```python
from build123d import *

# Parameters (mm, degrees)
SKETCH3_R           = 0.6
BOSS_EXTRUDE1_DEPTH = 2.5
CIRPATTERN1_COUNT   = 4
BOSS_EXTRUDE2_DEPTH = 1


with BuildPart() as part:
    # Sketch2 → Revolve1 (revolve)
    with BuildSketch(Plane(origin=(0, 0, 0), x_dir=(0, 0, -1), z_dir=(1, 0, 0))):
        Polygon((0, 8.815), (0, 10), (-1.5, 10), (-1.5, 7.74), (5, 7.74), (5, 5.555), (0.5, 5.555), (0.5, 0), (11.17, 0), (11.17, 7.25), (10.130849194, 7.25), (9, 8.815), align=None)
    revolve(axis=Axis((0, 0, 11.357142857), (0, 0, -1)))

    # Sketch3 → Boss-Extrude1 (add)
    with BuildSketch(Plane(origin=(0, 0, -11.17), x_dir=(-1, 0, 0), z_dir=(0, 0, -1))):
        with Locations((1.71395454, 3.773699623)):
            Circle(SKETCH3_R)
        with Locations((1.71395454, 1.968598852)):
            Circle(SKETCH3_R)
        with Locations((3.52115951, 1.968598852)):
            Circle(SKETCH3_R)
    boss_extrude1 = extrude(amount=BOSS_EXTRUDE1_DEPTH)

    # CirPattern1: Boss-Extrude1 ×4 about axis
    cirpattern1_axis = Axis((0, 0, 0), (0, 0, 1))
    for i in range(1, CIRPATTERN1_COUNT):
        add(boss_extrude1.rotate(cirpattern1_axis, i * 360 / CIRPATTERN1_COUNT))

    # Sketch5 → Boss-Extrude2 (add)
    with BuildSketch(Plane(origin=(0, 0, 0), x_dir=(-1, 0, 0), z_dir=(0, 0, -1))):
        with BuildLine():
            Line((-0.71671494, 9.974282916), (-0.71671494, 8.78581497))
            ThreePointArc((-0.71671494, 8.78581497), (0, 8.815), (0.71671494, 8.78581497))
            Line((0.71671494, 8.78581497), (0.71671494, 9.974282916))
            ThreePointArc((0.71671494, 9.974282916), (0, 10), (-0.71671494, 9.974282916))
        make_face()
    extrude(amount=BOSS_EXTRUDE2_DEPTH)


solid = part.part
```
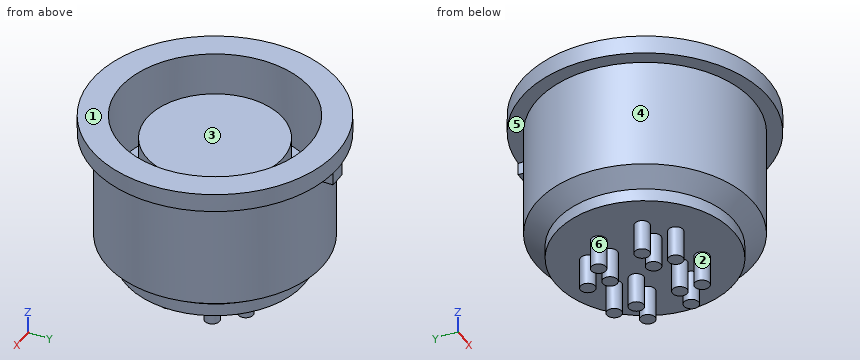
Part model, mm, in its own coordinate system. Face numbers are marked on the shaded views. A direction names the side the tool comes from. Round coordinates to 2 decimals unless told otherwise and drop trailing zeros. Loops run counter-clockwise (first coordinate to the right, second up) from the corner with the lowest first, then second, coordinate; pieces in that order, holes last. Notation, with made-up numbers: (48, 40) -> (58, 40) arc R30 cw to (58, 73) -> close; hole circle Ø4 at (11, 12.5). An arc over 180 degrees is marked (long way). Use one line per item in the form item = value. Start each with the question number.
Item 1: Two-plate mould, pull along Y, no slides. Class the marked faces 4, 5 and 6: released by +Y, released by -Y, zero draft, split by the parting line, or undercut.
Item 2: Band-saw the part on C-C (y = 0). List the corners of the cut face in (x, z) (3 decimals), plus the area to 3 significant figures.
Item 3: Drill centre lines: line 1 along X through (y, z) = (0, -1.75) (3 decimals); line 2 along Z through (x, y) = (-2.75, -1.75); line 3 along X through (y, z) = (-6.75, -3.5). Where is each one in solid material? Low to high.
Item 4: Band-saw the part on A-A (x = 0). List the corners of the cut face in (y, z) (3 decimals), plus the area to 3 significant figures.
Item 5: Band-saw the part on D-D (z = -11.5). Give the number of separate pieces and of enclosed holes in the cut face, plus the area to 3 significant figures.
Item 6: Tool access for the marked faces 1, 2 and 3: list every direction of +Z, -Z, +X, -X, +Y, -Y with a clear straight run to the whole face (end or side of a thin tool).
Item 7: Band-saw the part on B-B (z = -2.5). List the corners of the cut face in (x, y) (3 decimals), plus the area to 3 significant figures.
Item 8: Drop flat-ended pins along their axis: pin 1 Ø3 at (x, z) = (-2, -1) entering from -Y; pin 2 Ø1 at (y, z) = (-4.5, -9) entering from +X; pin 3 Ø10 at (x, y) = (-6, 2.5) entering from +Z; pin 4 Ø12 at (x, y) = (1, 1) entering from +Z. Give the stop position or say it passes through.
Data:
q1.face_4 = split by the parting line
q1.face_5 = zero draft
q1.face_6 = undercut
q2.outline = (-10, 0) -> (-8.815, 0) -> (-8.815, -9) -> (-7.25, -10.131) -> (-7.25, -11.17) -> (7.25, -11.17) -> (7.25, -10.131) -> (8.815, -9) -> (8.815, 0) -> (10, 0) -> (10, 1.5) -> (7.74, 1.5) -> (7.74, -5) -> (5.555, -5) -> (5.555, -0.5) -> (-5.555, -0.5) -> (-5.555, -5) -> (-7.74, -5) -> (-7.74, 1.5) -> (-10, 1.5) -> close
q2.area = 171 mm^2
q3.line_1 = -8.815 to -7.74, -5.555 to 5.555, 7.74 to 8.815
q3.line_2 = -11.17 to -0.5
q3.line_3 = -5.67 to -3.79, 3.79 to 5.67
q4.outline = (-10, 0) -> (-8.815, 0) -> (-8.815, -9) -> (-7.25, -10.131) -> (-7.25, -11.17) -> (7.25, -11.17) -> (7.25, -10.131) -> (8.815, -9) -> (8.815, -1) -> (10, -1) -> (10, 1.5) -> (7.74, 1.5) -> (7.74, -5) -> (5.555, -5) -> (5.555, -0.5) -> (-5.555, -0.5) -> (-5.555, -5) -> (-7.74, -5) -> (-7.74, 1.5) -> (-10, 1.5) -> close
q4.area = 172 mm^2
q5.separate_pieces = 12
q5.enclosed_holes = 0
q5.area = 13.6 mm^2
q6.face_1 = +Z, +X, -X, +Y, -Y
q6.face_2 = -Z
q6.face_3 = +Z
q7.outline = circle Ø17.63 at (0, 0); circle Ø11.11 at (0, 0); hole circle Ø15.48 at (0, 0)
q7.area = 153 mm^2
q8.pin_1 = -9.96
q8.pin_2 = 7.86
q8.pin_3 = 1.5
q8.pin_4 = -0.5
